```python
from build123d import *

# Parameters (mm, degrees)
SKETCH1_R           = 11
BOSS_EXTRUDE1_DEPTH = 40
BOSS_EXTRUDE2_DEPTH = 8
FILLET1_R           = 2


with BuildPart() as part:
    # Sketch1 → Boss-Extrude1 (new body)
    with BuildSketch(Plane.XY):
        Circle(SKETCH1_R)
    extrude(amount=-BOSS_EXTRUDE1_DEPTH)

    # Sketch2 → Boss-Extrude2 (add)
    with BuildSketch(Plane(origin=(0, 0, -40), x_dir=(-1, 0, 0), z_dir=(0, 0, -1))):
        Polygon((6.350852961, 11), (-6.350852961, 11), (-12.701705922, 0), (-6.350852961, -11), (6.350852961, -11), (12.701705922, 0), align=None)
    extrude(amount=BOSS_EXTRUDE2_DEPTH)

    # Sketch6 → Revolve1 (revolve)
    with BuildSketch(Plane(origin=(0, 0, 0), x_dir=(0, 0, -1), z_dir=(1, 0, 0)), mode=Mode.PRIVATE) as revolve1_sk:
        Polygon((48, 6.86), (66, 6.297503336), (66, 2), (48, 2), align=None)
    revolve(revolve1_sk.sketch.rotate(Axis((0, 0, 0), (0, 0, 1)), 90), axis=Axis((0, 0, 0), (0, 0, 1)))

    # Fillet1
    fillet1_edges = [part.edges().sort_by_distance(p)[0] for p in [
        (-11, 0, 0),
    ]]
    fillet(fillet1_edges, radius=FILLET1_R)


solid = part.part
```
For this review, take the finished solid that the model builds, in its own axes (mm). A direction names the side the tool comes from. Round coordinates to 2 decimals unless told otherwise and drop trailing zeros. Write each loop counter-clockwise with the first axis right and the second up, starting at its lowest first coordinate (ties: lowest second). Pieces come first, ordered by that corner, then holes. Notation, with made-up numbers: (82, 46.25) - (111, 46.25) arc R17 cw to (111, 69.25) - close; hole circle Ø11 at (33.5, -14). An arc over 180 degrees is marked (long way). Answer as CSV lines item,"result". Start each with the question number.
(1) Machinability: for faces 1 (the flat face through (5, 10, -40)), 2 (the cylindrical face through (-2.38, -10.74, -20.73)), 3 (the flat face through (-6, 10, -40)), 4 (the flat face through (5, -10, -40)), 5 (the flat face through (-5, 5, -48)), which of the approach directions +Z, -Z, +X, -X, +Y, -Y give a long, thin tool a straight path to every point of the face, cutting with its end or side? Answer none if there is none.
(2) For line 1 (Y direction, x = 0, z = -54.5); line 2 (Z direction, x = -7.25, y = -1.75); line 3 (Y direction, x = 0, z = -55), list the stretches that pass through material, from the lowest coordinate up.
(3) Mouldability with a two-part tool opening along Y and no side actions: class faces 6 (the flat face through (11.4, 0, -40)), 7 (the flat face through (0, 0, -48)), 8 (the flat face through (0, -11, -44)) as +Y half, -Y half, draft (parallel to the pull), parting line (faces both ways), or undercut.
(4) Add section B-B, the plane z = -49. State the section outline as (x, y) points, plus the area to 3 significant figures.
(5) Add section A-A, the plane z = -14.5. State the section outline as (x, y) points.
(6) For pin 1 (3 mm diameter, centred on x = 0, y = 0, fed in from +Z); pin 2 (3 mm diameter, centred on x = 9.5, y = 6, fed in from -Z); pin 3 (6 mm diameter, centred on x = -7, z = -26, fed in from -Y); pin 4 (1 mm diameter, centred on x = -11, y = 0, fed in from +Z), all flat-tipped, find the tip position at first contact; note any pin that passes through.
From the geometry:
1,face 1,"+Z, +X, +Y"
1,face 2,"+Z"
1,face 3,"+Z, -X, +Y"
1,face 4,"+Z, +X, -Y"
1,face 5,"-Z"
2,line 1,"y = -6.66 to -2, 2 to 6.66"
2,line 2,"z = -48 to 0"
2,line 3,"y = -6.64 to -2, 2 to 6.64"
3,face 6,"draft"
3,face 7,"undercut"
3,face 8,"-Y half"
4,outline,"circle Ø13.66 at (0, 0); hole circle Ø4 at (0, 0)"
4,area,"134 mm²"
5,outline,"circle Ø22 at (0, 0)"
6,pin 1,"stops at z = 0"
6,pin 2,"stops at z = -48"
6,pin 3,"stops at y = -10.25"
6,pin 4,"stops at z = -0.68"
